```python
from build123d import *

# Parameters (mm, degrees)
F0_W     = 489.3
F0_H     = 44.5
F1_DEPTH = 483
F2_W     = 37.4
F2_H     = 44.5
F3_DEPTH = 475
F5_DEPTH = 8
F8_R     = 3.175


with BuildPart() as f1:
    # F0 (on Front) → F1 (new body)
    with BuildSketch(Plane.XZ):
        Rectangle(F0_W, F0_H)
    extrude(amount=-F1_DEPTH)

    # F2 (on face) → F3 (cut)
    with BuildSketch(Plane(origin=(0, 483, 0), x_dir=(-1, 0, 0), z_dir=(0, 1, 0))):
        with Locations((-225.95, 0)):
            Rectangle(F2_W, F2_H)
        with Locations((225.95, 0)):
            Rectangle(F2_W, F2_H)
    extrude(amount=-F3_DEPTH, mode=Mode.SUBTRACT)

    # F4 (on face) → F5 (cut, through all)
    with BuildSketch(Plane.XZ):
        with BuildLine():
            Line((-235.325, 12.725), (-228.975, 12.725))
            ThreePointArc((-228.975, 12.725), (-225.8, 15.9), (-228.975, 19.075))
            Line((-228.975, 19.075), (-235.325, 19.075))
            ThreePointArc((-235.325, 19.075), (-238.5, 15.9), (-235.325, 12.725))
        make_face()
        with BuildLine():
            Line((-228.975, -12.725), (-235.325, -12.725))
            ThreePointArc((-235.325, -12.725), (-238.5, -15.9), (-235.325, -19.075))
            Line((-235.325, -19.075), (-228.975, -19.075))
            ThreePointArc((-228.975, -19.075), (-225.8, -15.9), (-228.975, -12.725))
        make_face()
        with BuildLine():
            Line((235.325, 19.075), (228.975, 19.075))
            ThreePointArc((228.975, 19.075), (225.8, 15.9), (228.975, 12.725))
            Line((228.975, 12.725), (235.325, 12.725))
            ThreePointArc((235.325, 12.725), (238.5, 15.9), (235.325, 19.075))
        make_face()
        with BuildLine():
            Line((235.325, -12.725), (228.975, -12.725))
            ThreePointArc((228.975, -12.725), (225.8, -15.9), (228.975, -19.075))
            Line((228.975, -19.075), (235.325, -19.075))
            ThreePointArc((235.325, -19.075), (238.5, -15.9), (235.325, -12.725))
        make_face()
    extrude(amount=-F5_DEPTH, mode=Mode.SUBTRACT)

    # F9: sweep along a path in F7
    with BuildLine(Plane.YZ.offset(-228.6)) as f9_path:
        Line((0, 15.9), (-23.15, 15.9))
        ThreePointArc((-23.15, 15.9), (-27.6401280605, 14.0401280605), (-29.5, 9.55))
        Line((-29.5, 9.55), (-29.5, -9.55))
        ThreePointArc((-29.5, -9.55), (-27.6401280605, -14.0401280605), (-23.15, -15.9))
        Line((-23.15, -15.9), (0, -15.9))
    # F8 (on face) → F9 (sweep)
    with BuildSketch(Plane.XZ):
        with Locations((-221.79, 15.9)):
            Circle(F8_R)
    sweep(path=f9_path.line)

    # F10: F1 across plane


with BuildPart() as f1_1:
    add(f1.part)
    add(f1.part.mirror(Plane.YZ))


solid = f1_1.part
```
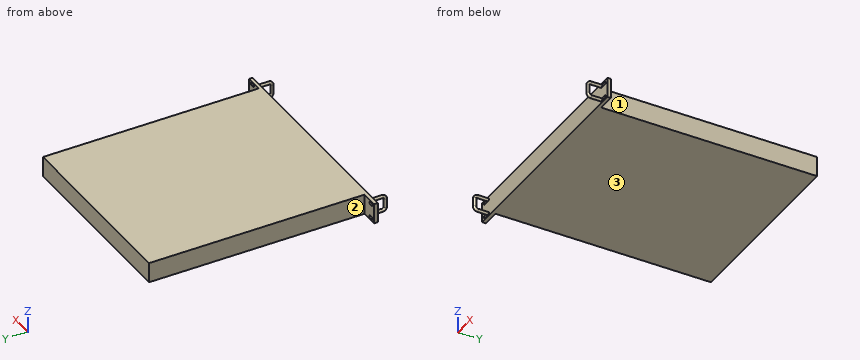
Work out the finished part from the listing and answer in its coordinate system (mm). Face numbers are marked on the shaded views. A direction names the side the tool comes from. Give positions to 0.01 mm unless a question says otherwise; leave off trailing zeros. Order: outer loops, then holes, each group sorted by start corner. A loop starts at its lowest first (then second) coordinate and runs counter-clockwise, first axis right, second up. Notation, with made-up numbers: M 20,7 L 55,7 A20 cw 55,27 Z; hole C 72,47 d2. An arc over 180 degrees is marked long. Return JSON: item names as keys, results as strings.
1) Section A-A, the plane z = -2.5 is taken. Write down the section's boundary in (x, y) (3 decimals).
Resolved:
{"outline": "M -244.65,0 L 244.65,0 L 244.65,8 L 207.25,8 L 207.25,483 L -207.25,483 L -207.25,8 L -244.65,8 Z; C -221.79,-29.5 d6.35; C 221.79,-29.5 d6.35"}
2) Each of these flat-tipped pins is pushed along its axis until it touches: pin 1 (18.5 mm diameter, centred on x = 235, z = -4, fed in from +Y); pin 2 (10 mm diameter, centred on y = 148.5, z = -1, fed in from +X); pin 3 (12 mm diameter, centred on x = 118, z = -16, fed in from -Y). Where does it stop, or does it pass through?
Resolved:
{"pin 1": "y = 8", "pin 2": "x = 207.25", "pin 3": "y = 0"}
3) Section C-C, the plane y = 66 is taken. Write down the section's boundary in (x, z).
Resolved:
{"outline": "M -207.25,-22.25 L 207.25,-22.25 L 207.25,22.25 L -207.25,22.25 Z"}
4) A tool of negligible diameter and unlimited length cuts with its end or side. For the marked faces 1, 2 and 3, from which of +Z, -Z, +X, -X, +Y, -Y can it reach the whole face along a straight path? Write none if from no direction.
Resolved:
{"face 1": "+Z, -Z, +X, +Y", "face 2": "+Z, -Z, -X, +Y", "face 3": "-Z, +X, -X, +Y, -Y"}
5) Section B-B, the plane x = 88.5 is taken. Write down the section's boundary in (y, z).
Resolved:
{"outline": "M 0,-22.25 L 483,-22.25 L 483,22.25 L 0,22.25 Z"}
6) Straight lines are drawn through the part: line 1 along X through (y, z) = (402, 15); line 2 along Y through (x, z) = (-96, 5.5). For each, find the intervals that lie inside material, in ascending order. Write a range as [from, to].
Resolved:
{"line 1": "[-207.25, 207.25]", "line 2": "[0, 483]"}
